Autodesk Inventor part; units mm, degrees
ref_plane "YZ Plane" through (0, 0, 0) normal (1, 0, 0) x (0, 1, 0)
ref_plane "XZ Plane" through (0, 0, 0) normal (0, 1, 0) x (-1, 0, 0)
ref_plane "XY Plane" through (0, 0, 0) normal (0, 0, 1) x (1, 0, 0)
sketch "Sketch1" plane through (0, 0, 0) normal (0, 0, 1) x (1, 0, 0)
  line L0 (-33.02, -22.225) -> (33.02, -22.225)
  line L1 (33.02, -22.225) -> (33.02, 22.225)
  line L2 (33.02, 22.225) -> (-33.02, 22.225)
  line L3 (-33.02, 22.225) -> (-33.02, -22.225)
  line L4 (-33.02, -22.225) -> (33.02, 22.225) construction
  line L5 (33.02, -22.225) -> (-33.02, 22.225) construction
  point P0 (0, 0)
  dimension "d0" = 66.04
  dimension "d1" = 44.45
extrude "Extrusion1" add sketch "Sketch1" along normal mid plane 8.7376
sketch "Sketch2" plane through (0, 0, 4.3688) normal (0, 0, 1) x (1, 0, 0)
  line L0 (-33.02, -22.225) -> (33.02, -22.225)
  line L1 (33.02, -22.225) -> (33.02, 22.225)
  line L2 (33.02, 22.225) -> (-33.02, 22.225)
  line L3 (-33.02, 22.225) -> (-33.02, -22.225)
  circle A0 centre (0, 0) radius 17.4625
  dimension "d4" = 34.925
hole "Hole1" at (0, 0, 4.3688) direction (0, 0, -1) diameter 34.925 end through all
sketch "Sketch3" plane through (0, 0, 4.3688) normal (0, 0, 1) x (1, 0, 0)
  circle A0 centre (0, 0) radius 17.4625
  line L0 (-33.02, -22.225) -> (33.02, -22.225)
  line L1 (33.02, -22.225) -> (33.02, 22.225)
  line L2 (33.02, 22.225) -> (-33.02, 22.225)
  line L3 (-33.02, 22.225) -> (-33.02, -22.225)
  circle A1 centre (-25.4, 0) radius 2.54
  line L4 (0, 22.225) -> (0, -22.225) construction
  circle A2 centre (25.4, 0) radius 2.54
  dimension "d12" = 5.08
  dimension "d13" = 7.62
hole "Hole2" at (-25.4, 0, 4.3688) at (25.4, 0, 4.3688) direction (0, 0, -1) diameter 5.08 end through all
properties part number "Tapered Roller Bearing Housing" material "Aluminum 6061"
CAD build for the part. Positions are in the model's coordinates, mm. Coordinates: 2 decimals unless noted, no trailing zeros. Loops run counter-clockwise (first coordinate to the right, second up) from the corner with the lowest first, then second, coordinate; pieces in that order, holes last. Notation, with made-up numbers: (-11, 73.25) -> (28, 73.25) arc R8 cw to (28, 84.25) -> close; hole circle Ø6 at (80.5, 64). An arc over 180 degrees is marked (long way). One line per item, written item: value.
1. Pull direction X, two halves, no side cores. Call faces 1 (the face through (33.02, 0, 0)), 2 (the face through (-27.92, 0.33, -0.06)), 3 (the face through (0, 22.225, 0)): pulls with the +X half, pulls with the -X half, needs draft (parallel to the pull), parting line crosses it, or undercut.
Answers:
face 1: pulls with the +X half
face 2: undercut
face 3: needs draft
2. Slice it at C-C on x = -25.4. Write the cut outline in (y, z) (3 decimals).
Answers:
outline: (-22.225, -4.369) -> (-2.54, -4.369) -> (-2.54, 4.369) -> (-22.225, 4.369) -> close; (2.54, -4.369) -> (22.225, -4.369) -> (22.225, 4.369) -> (2.54, 4.369) -> close
3. Slice it at A-A on y = 0. Write the cut outline in (x, z).
Answers:
outline: (-33.02, -4.37) -> (-27.94, -4.37) -> (-27.94, 4.37) -> (-33.02, 4.37) -> close; (-22.86, -4.37) -> (-17.46, -4.37) -> (-17.46, 4.37) -> (-22.86, 4.37) -> close; (17.46, -4.37) -> (22.86, -4.37) -> (22.86, 4.37) -> (17.46, 4.37) -> close; (27.94, -4.37) -> (33.02, -4.37) -> (33.02, 4.37) -> (27.94, 4.37) -> close
4. Slice it at B-B on z = -3.5. Write the cut outline in (x, y) (1 decimal).
Answers:
outline: (-33, -22.2) -> (33, -22.2) -> (33, 22.2) -> (-33, 22.2) -> close; hole circle Ø5.1 at (-25.4, 0); hole circle Ø34.9 at (0, 0); hole circle Ø5.1 at (25.4, 0)
5. Drill centre lines: line 1 (X direction, y = 0, z = 2.75); line 2 (Y direction, x = 0, z = 0.75) (1 decimal); line 3 (Y direction, x = -25.4, z = 0) (3 decimals). Where is each one in solid material? Low to high. Write a range as [from, to].
Answers:
line 1: x = [-33.02, -27.94], [-22.86, -17.46], [17.46, 22.86], [27.94, 33.02]
line 2: y = [-22.2, -17.5], [17.5, 22.2]
line 3: y = [-22.225, -2.54], [2.54, 22.225]
6. Slice it at D-D on y = 7.5. Write the cut outline in (x, z).
Answers:
outline: (-33.02, -4.37) -> (-15.77, -4.37) -> (-15.77, 4.37) -> (-33.02, 4.37) -> close; (15.77, -4.37) -> (33.02, -4.37) -> (33.02, 4.37) -> (15.77, 4.37) -> close
